```python
from build123d import *

# Parameters (mm, degrees)
F1_DEPTH = 4.318
F0_W     = 74.9314
F0_H     = 67.056
F2_DEPTH = 5.08
F3_DEPTH = 3.556
F4_R     = 2.032
F5_R     = 7.62
F6_R     = 5.08


# Not quite as in the source:
# - a feature names something its author has since deleted; it is built from what else it names


with BuildPart() as f1:
    # F0 (on Top) → F1 (new body)
    with BuildSketch(Plane.XY):
        with BuildLine():
            Line((2.8111794461, 24.3078), (2.8111794461, 41.656))
            Line((2.8111794461, 41.656), (-7.0454205539, 41.656))
            Line((-7.0454205539, 41.656), (-7.0454205539, 37.6428))
            Line((-7.0454205539, 37.6428), (-21.6488205539, 37.6428))
            Line((-21.6488205539, 37.6428), (-21.6488205539, 20.193))
            Line((-21.6488205539, 20.193), (-36.7380205539, 20.193))
            Line((-36.7380205539, 20.193), (-36.7380205539, 6.731))
            Line((-36.7380205539, 6.731), (-30.5658055774, 6.731))
            ThreePointArc((-30.5658055774, 6.731), (-26.9316083266, 16.200428444), (-18.8310205539, 10.0965))
            ThreePointArc((-18.8310205539, 10.0965), (-19.0770921098, 8.3459122272), (-19.7962355303, 6.731))
            Line((-19.7962355303, 6.731), (-13.6188205539, 6.731))
            Line((-13.6188205539, 6.731), (-13.6188205539, 29.2354))
            Line((-13.6188205539, 29.2354), (-6.0548205539, 29.2354))
            Line((-6.0548205539, 29.2354), (-6.0548205539, 24.3078))
            Line((-6.0548205539, 24.3078), (2.8111794461, 24.3078))
        make_face()
    extrude(amount=F1_DEPTH)

    # F0 (on Top) → F2 (join)
    with BuildSketch(Plane.XY):
        with Locations((-21.9545205539, 20.828)):
            Rectangle(F0_W, F0_H)
        Polygon((-7.0454205539, 41.656), (2.8111794461, 41.656), (2.8111794461, 24.3078), (-6.0548205539, 24.3078), (-6.0548205539, 29.2354), (-13.6188205539, 29.2354), (-13.6188205539, 6.731), (1.3111794461, 6.731), (1.3111794461, 0), (-46.7202205539, 0), (-46.7202205539, 6.731), (-36.7380205539, 6.731), (-36.7380205539, 20.193), (-21.6488205539, 20.193), (-21.6488205539, 37.6428), (-7.0454205539, 37.6428), align=None, mode=Mode.SUBTRACT)
    extrude(amount=F2_DEPTH)

    # F0 (on Top) → F3 (join)
    with BuildSketch(Plane.XY):
        with BuildLine():
            Line((1.3111794461, 6.731), (-13.6188205539, 6.731))
            Line((-13.6188205539, 6.731), (-19.7962355303, 6.731))
            ThreePointArc((-19.7962355303, 6.731), (-25.1810205539, 3.7465), (-30.5658055774, 6.731))
            Line((-30.5658055774, 6.731), (-36.7380205539, 6.731))
            Line((-36.7380205539, 6.731), (-46.7202205539, 6.731))
            Line((-46.7202205539, 6.731), (-46.7202205539, 0))
            Line((-46.7202205539, 0), (1.3111794461, 0))
            Line((1.3111794461, 0), (1.3111794461, 6.731))
        make_face()
    extrude(amount=F3_DEPTH)

    # F4
    f4_edges = [f1.edges().sort_by_distance(p)[0] for p in [
        (-7.045421, 37.6428, 4.699),
        (-13.618821, 29.2354, 4.699),
        (-21.648821, 20.193, 4.699),
        (-13.618821, 6.731, 4.699),
        (-36.738021, 6.731, 4.699),
        (-6.054821, 29.2354, 4.699),
    ]]
    fillet(f4_edges, radius=F4_R)

    # F5
    f5_edges = [f1.edges().sort_by_distance(p)[0] for p in [
        (-36.738021, 20.193, 4.699),
    ]]
    fillet(f5_edges, radius=F5_R)

    # F6
    f6_edges = [f1.edges().sort_by_distance(p)[0] for p in [
        (15.511179, -12.7, 2.54),
        (15.511179, 54.356, 2.54),
        (-59.420221, 54.356, 2.54),
        (-59.420221, -12.7, 2.54),
    ]]
    fillet(f6_edges, radius=F6_R)


solid = f1.part
```
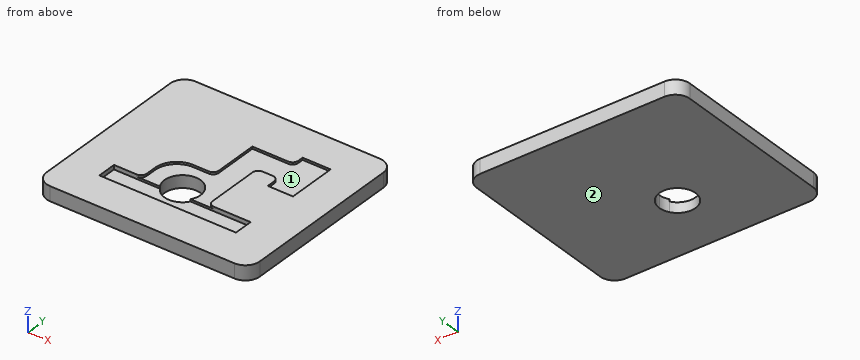
CAD build for the part. Positions are in the model's coordinates, mm. Face numbers are marked on the shaded views. Give positions to 0.01 mm unless a question says otherwise; leave off trailing zeros. Loops run counter-clockwise (first coordinate to the right, second up) from the corner with the lowest first, then second, coordinate; pieces in that order, holes last. Notation, with made-up numbers: (23.25, 50.25) -> (32.25, 50.25) arc R24 cw to (32.25, 64.25) -> close; hole circle Ø10 at (88.25, -21). An arc over 180 degrees is marked (long way). Use a Markdown table: item, result.
1. Wall check: L1, parallel to Y at x = -9, z = 4.75; L2, parallel to X at y = 25.5, z = 4.85; L3, parallel to X at y = 36.5, z = 4.4. Give the ranges that are in metal, low to high. Write a range as [from, to].
Check result:
| item | result |
|---|---|
| L1 | y = [-12.7, 0], [6.73, 29.24], [37.64, 54.36] |
| L2 | x = [-59.42, -21.65], [-13.62, -6.05], [2.81, 15.51] |
| L3 | x = [-59.42, -21.65], [2.81, 15.51] |
2. Flat gauge pins, fed straight in: pin 1 (10 mm diameter, centred on x = -38.5, y = 3, fed in from +Z); pin 2 (3.5 mm diameter, centred on x = -24, y = 4, fed in from +Z). Where does each tip first touch, or does it go through?
Check result:
| item | result |
|---|---|
| pin 1 | stops at z = 5.08 |
| pin 2 | stops at z = 3.56 |
3. Slice it at A-A (z = 1.05). List the corners of the cut face in (x, y).
Check result:
| item | result |
|---|---|
| outline | (-59.42, -7.62) arc R5.08 ccw to (-54.34, -12.7) -> (10.43, -12.7) arc R5.08 ccw to (15.51, -7.62) -> (15.51, 49.28) arc R5.08 ccw to (10.43, 54.36) -> (-54.34, 54.36) arc R5.08 ccw to (-59.42, 49.28) -> close; hole circle Ø12.7 at (-25.18, 10.1) |
4. Slice it at B-B (x = -34.5). List the corners of the cut face in (y, z), plus the area to 3 significant figures.
Check result:
| item | result |
|---|---|
| outline | (-12.7, 0) -> (54.36, 0) -> (54.36, 5.08) -> (17.97, 5.08) -> (17.97, 4.32) -> (6.73, 4.32) -> (6.73, 3.56) -> (0, 3.56) -> (0, 5.08) -> (-12.7, 5.08) -> close |
| area | 322 mm^2 |
5. Mould opens along Y. For the marked faces 1 and 2 say: pulls with the +Y half, pulls with the -Y half, needs draft (parallel to the pull), parting line crosses it, or undercut.
Check result:
| item | result |
|---|---|
| face 1 | undercut |
| face 2 | needs draft |
